Input: part model. Units: mm. Frame: model coordinates. A direction names the side the tool comes from. Give positions to 0.01 mm unless a question says otherwise; leave off trailing zeros. Loops run counter-clockwise (first coordinate to the right, second up) from the corner with the lowest first, then second, coordinate; pieces in that order, holes last. Notation, with made-up numbers: (-9, -31.75) -> (32, -31.75) arc R11 ccw to (32, -11.75) -> close; hole circle Ø8 at (-36.75, 25.25). An arc over 180 degrees is marked (long way). One line per question, with ' | ' between items.
Autodesk Inventor part; units mm, degrees
ref_plane "РабПлоскость2" through (0, 0, -38.7685) normal (0, 0, 1) x (-1, 0, 0)
ref_plane "YZ Plane" through (0, 0, 0) normal (1, 0, 0) x (0, 1, 0)
ref_plane "XZ Plane" through (0, 0, 0) normal (0, 1, 0) x (-1, 0, 0)
ref_plane "РабПлоскость2" through (0, 0, -38.7685) normal (0, 0, 1) x (-1, 0, 0)
sketch "Эскиз2" plane through (0, 0, -38.7685) normal (0, 0, 1) x (-1, 0, 0)
  line L0 (0, 0) -> (0, -166.5002) construction
  circle A0 centre (72.2445, -74.8113) radius 26 construction
  circle A1 centre (100.9108, -25.1599) radius 26 construction
  circle A2 centre (-72.2445, -74.8113) radius 26 construction
  circle A3 centre (-100.9108, -25.1599) radius 26 construction
  circle A4 centre (72.2445, -74.8113) radius 26.25
  circle A5 centre (100.9108, -25.1599) radius 26.25
  circle A6 centre (-72.2445, -74.8113) radius 26.25
  circle A7 centre (-100.9108, -25.1599) radius 26.25
  circle A8 centre (0, 0) radius 132.5
  circle A9 centre (0, 0) radius 75.5
  circle A10 centre (100.9108, -25.1599) radius 28.5
  circle A11 centre (-100.9108, -25.1599) radius 28.5
  circle A12 centre (0, 0) radius 120.5
  line L1 (0, 0) -> (-34.2935, -127.9852)
  line L2 (0, 0) -> (34.2935, -127.9852)
  point P0 (-128.5642, -32.0547)
  point P1 (128.5642, -32.0547)
  point P2 (73.2573, -18.2651)
  point P3 (-73.2573, -18.2651)
  point P4 (-31.1877, -116.3941)
  point P5 (31.1877, -116.3941)
  dimension "d0" = 52.5
  dimension "d2" = 151
  dimension "d5" = 30
  dimension "d6" = 12
extrude "Выдавливание1" add sketch "Эскиз2" along normal blind 6 contours A4 A12 A10 A8 L2 | A4 A12 L2 A9 A10 | A12 A5 A10 | A10 A12 A5 | A12 L1 A9 L2 | L1 A8 A11 A12 A6 | A12 A6 A11 A9 L1 | A11 A12 A7 | A11 A12 A7
properties part number "Диск_фиксатор"
1. Ray query, line 1 along X through (y, z) = (81, -33.8); line 2 along X through (y, z) = (90.5, -35.15); line 3 along Y through (x, z) = (84.5, -38.2). Return the intervals inside material, ascending. Write a range as from..to.
Determined:
line 1: x = -104.86..-97.75, -46.73..46.73, 97.75..104.86 | line 2: x = -96.78..-93.29, -51.2..51.2, 93.29..96.78 | line 3: y = 1.86..4.67, 45.65..51.6, 98.02..102.06
2. Section query C-C (x = 91.5). Output: boundary loops of the cut face in (y, z), then the cut area to 3 significant figures.
Determined:
outline: (-1.74, -38.77) -> (0.65, -38.77) -> (0.65, -32.77) -> (-1.74, -32.77) -> close; (49.66, -38.77) -> (56.97, -38.77) -> (56.97, -32.77) -> (49.66, -32.77) -> close; (92.65, -38.77) -> (95.83, -38.77) -> (95.83, -32.77) -> (92.65, -32.77) -> close | area: 77.3 mm2
3. Pin query (flat end, axial travel): P1, Ø1.5, axis at x = -57.5, z = -33.5, coming from the -Y side. Return the tip coordinate at first contact, or that it passes through.
Determined:
P1: stops at y = 48.03
4. Pull-direction query (Y, two-part tool) for faces 1 (the flat face through (1, 86, -38.768)), 2 (the cylindrical face through (-97.28, 82.7, -35.81)), 3 (the flat face through (32.72, 122.11, -35.81)); classes: pulls with the +Y half, pulls with the -Y half, needs draft (parallel to the pull), parting line crosses it, or undercut.
Determined:
face 1: needs draft | face 2: undercut | face 3: pulls with the +Y half
5. Reachability of faces 4 (the flat face through (-32.72, 122.11, -35.81)), 5 (the cylindrical face through (-95.2, 92.16, -35.81)) from +Z, -Z, +X, -X, +Y, -Y: full face, straight path, thin tool, end or side. Return the list, or none.
Determined:
face 4: +Z, -Z, +Y | face 5: +Z, -Z, -X, +Y
6. Section query B-B (y = 43). Output: boundary loops of the cut face in (x, z), then the cut area to 3 significant figures.
Determined:
outline: (-125.33, -38.77) -> (-120.17, -38.77) -> (-120.17, -32.77) -> (-125.33, -32.77) -> close; (-81.65, -38.77) -> (-62.06, -38.77) -> (-62.06, -32.77) -> (-81.65, -32.77) -> close; (62.06, -38.77) -> (81.65, -38.77) -> (81.65, -32.77) -> (62.06, -32.77) -> close; (120.17, -38.77) -> (125.33, -38.77) -> (125.33, -32.77) -> (120.17, -32.77) -> close | area: 297 mm2
7. Section query A-A (x = 56). Output: boundary loops of the cut face in (y, z).
Determined:
outline: (50.64, -38.77) -> (54.19, -38.77) -> (54.19, -32.77) -> (50.64, -32.77) -> close; (95.43, -38.77) -> (120.08, -38.77) -> (120.08, -32.77) -> (95.43, -32.77) -> close
